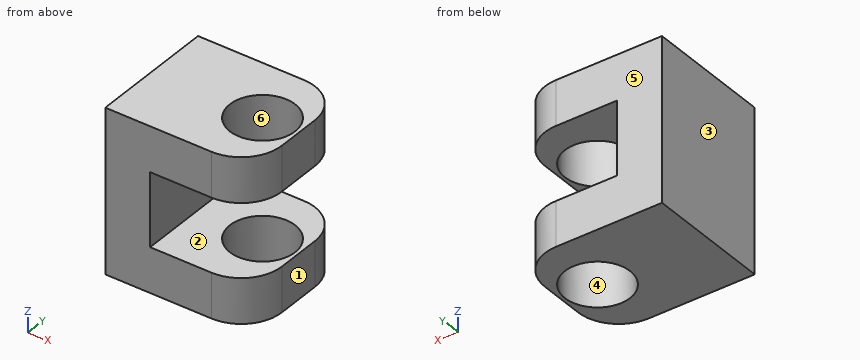
```python
from build123d import *

# Parameters (mm, degrees)
F0_W     = 25
F0_H     = 11
F0_W_2   = 11
F0_H_2   = 18
F1_DEPTH = 31
F3_D     = 16
F4_R     = 10


with BuildPart() as f1:
    # F0 (on Front) → F1 (new body)
    with BuildSketch(Plane.XZ):
        with Locations((5.5, 34.5)):
            Rectangle(F0_W, F0_H)
        with Locations((-12.5, 34.5)):
            Rectangle(F0_W_2, F0_H)
        with Locations((-12.5, 20)):
            Rectangle(F0_W_2, F0_H_2)
        with Locations((5.5, 5.5)):
            Rectangle(F0_W, F0_H)
        with Locations((-12.5, 5.5)):
            Rectangle(F0_W_2, F0_H)
    extrude(amount=F1_DEPTH)

    # F3 (through all)
    with Locations(Plane(origin=(0, 0, 0), x_dir=(1, 0, 0), z_dir=(0, 0, -1))):
        with Locations((9.1674635187, 15.4794855043)):
            Hole(F3_D / 2)

    # F4
    f4_edges = [f1.edges().sort_by_distance(p)[0] for p in [
        (18, 0, 5.5),
        (18, 0, 34.5),
        (18, -31, 5.5),
        (18, -31, 34.5),
    ]]
    fillet(f4_edges, radius=F4_R)


solid = f1.part
```
Design review of the part built by this model. Coordinates are the model's own, in mm. Face numbers are marked on the shaded views. A direction names the side the tool comes from. Coordinates: 2 decimals unless noted, no trailing zeros. Order: outer loops, then holes, each group sorted by start corner. A loop starts at its lowest first (then second) coordinate and runs counter-clockwise, first axis right, second up. Notation, with made-up numbers: M 38,7 L 80,7 A3 ccw 80,12 Z; hole C 8,1.25 d4. An arc over 180 degrees is marked long. Answer as a JSON object with one key per item and string values. Group by question number.
1) Add section A-A, the plane x = 6.5. Write out the cut boundary in (y, z).
2) Tool access review of the marked faces 1 and 2: name each direction out of +Z, -Z, +X, -X, +Y, -Y from which nothing blocks a thin tool from reaching the whole face with its end or side.
3) Add section D-D, the plane z = 37. Write out the cut boundary in (x, y), then the cut area to 3 significant figures.
4) Wall thickness on L1, parallel to Z at x = 16, y = -8.5; L2, parallel to Y at x = 10, z = 32; L3, parallel to X at y = -11, z = 32: over which ranges is each line inside the solid? List them lowest first.
5) Mouldability with a two-part tool opening along Y and no side actions: class the marked faces 3, 4, 5 and 6 as pulls with the +Y half, pulls with the -Y half, needs draft (parallel to the pull), parting line crosses it, or undercut.
6) For pin 1 (5 mm diameter, centred on x = 12, z = 35.5, fed in from -Y); pin 2 (5.5 mm diameter, centred on y = -19.5, z = 22.5, fed in from +X), all flat-tipped, find the tip position at first contact; note any pin that passes through.
7) Add section C-C, the plane x = -3.5. Write out the cut boundary in (y, z).
8) Add section B-B, the plane y = -9.5. Write out the cut boundary in (x, z).
Computed values:
{
 "1": {"outline": "M -31,0 L -23.02,0 L -23.02,11 L -31,11 Z; M -31,29 L -23.02,29 L -23.02,40 L -31,40 Z; M -7.94,0 L 0,0 L 0,11 L -7.94,11 Z; M -7.94,29 L 0,29 L 0,40 L -7.94,40 Z"},
 "2": {"face 1": "+Z, -Z, +X, +Y, -Y", "face 2": "+X, +Y, -Y"},
 "3": {"outline": "M -18,-31 L 8,-31 A10 ccw 18,-21 L 18,-10 A10 ccw 8,0 L -18,0 Z; hole C 9.17,-15.48 d16", "area": "872 mm^2"},
 "4": {"L1": "z = 0 to 11, 29 to 40", "L2": "y = -30.8 to -23.44, -7.52 to -0.2", "L3": "x = -18 to 2.54, 15.8 to 18"},
 "5": {"face 3": "needs draft", "face 4": "undercut", "face 5": "pulls with the +Y half", "face 6": "undercut"},
 "6": {"pin 1": "stops at y = -30.89", "pin 2": "stops at x = -7"},
 "7": {"outline": "M -31,0 L 0,0 L 0,11 L -31,11 Z; M -31,29 L 0,29 L 0,40 L -31,40 Z"},
 "8": {"outline": "M -18,0 L 3.85,0 L 3.85,11 L -7,11 L -7,29 L 3.85,29 L 3.85,40 L -18,40 Z; M 14.48,0 L 17.99,0 L 17.99,11 L 14.48,11 Z; M 14.48,29 L 17.99,29 L 17.99,40 L 14.48,40 Z"}
}
